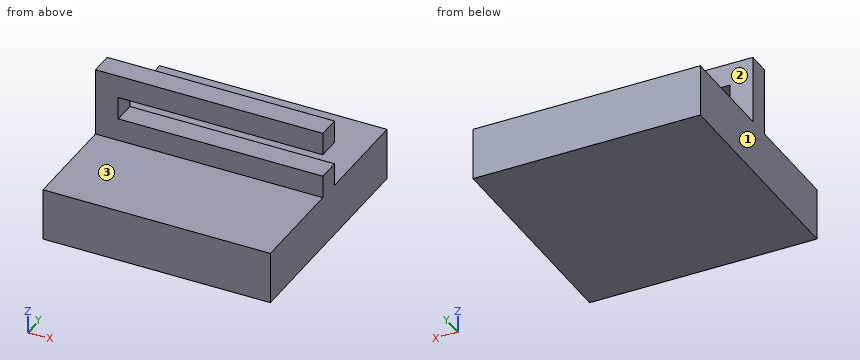
```python
from build123d import *

# Parameters (mm, degrees)
SKETCH1_W           = 100
SKETCH1_H           = 100
BOSS_EXTRUDE1_DEPTH = 23
SKETCH17_W          = 30
SKETCH17_H          = 10
BOSS_EXTRUDE2_DEPTH = 100
SKETCH18_W          = 90
SKETCH18_H          = 10
CUT_EXTRUDE1_DEPTH  = 126.833222958


with BuildPart() as part:
    # Sketch1 → Boss-Extrude1 (new body)
    with BuildSketch(Plane.XY):
        with Locations((50, 50)):
            Rectangle(SKETCH1_W, SKETCH1_H)
    extrude(amount=BOSS_EXTRUDE1_DEPTH)

    # Sketch17 → Boss-Extrude2 (add, through all)
    with BuildSketch(Plane(origin=(0, 0, 0), x_dir=(0, 0, -1), z_dir=(1, 0, 0))):
        with Locations((-38, 50)):
            Rectangle(SKETCH17_W, SKETCH17_H)
    extrude(amount=BOSS_EXTRUDE2_DEPTH)

    # Sketch18 → Cut-Extrude1 (cut, through all)
    with BuildSketch(Plane(origin=(0, 55, 0), x_dir=(1, 0, 0), z_dir=(0, 1, 0))):
        with Locations((55, -38)):
            Rectangle(SKETCH18_W, SKETCH18_H)
    extrude(amount=-CUT_EXTRUDE1_DEPTH, mode=Mode.SUBTRACT)


solid = part.part
```
Check sheet for the modelled part. Datum: model origin and axes. Units: mm. Face numbers are marked on the shaded views. A direction names the side the tool comes from. Give positions to 0.01 mm unless a question says otherwise; leave off trailing zeros. Write each loop counter-clockwise with the first axis right and the second up, starting at its lowest first coordinate (ties: lowest second). Pieces come first, ordered by that corner, then holes.
Item 1: Cross-section at B-B (y = 49). Enter the section's corners in (x, z), and give its area (3 significant figures).
Item 2: Cross-section at A-A (x = 20.5). Enter the section's corners in (y, z), and give its area (3 significant figures).
Item 3: Cross-section at C-C (z = 39). Enter the section's corners in (x, y).
Item 4: Gauge pin test, flat ends, axial feed: pin 1 (15 mm diameter, centred on x = 37, z = 42, fed in from -Y); pin 2 (22.5 mm diameter, centred on x = 61, y = 84, fed in from +Z); pin 3 (15 mm diameter, centred on x = 27.5, z = 36, fed in from +Y); pin 4 (5 mm diameter, centred on x = 51, z = 25, fed in from +Y). Record the tip position at first contact, or that the pin passes through.
Item 5: Cross-section at D-D (z = 26). Enter the section's corners in (x, y).
Item 6: Access from +Z, -Z, +X, -X, +Y, -Y to the whole of each face (thin tool, end or side, straight path). Record for the marked faces 1, 2 and 3.
Item 7: Scan lines: L1, parallel to Z at x = 20.5, y = 48.5; L2, parallel to Z at x = 32, y = 78; L3, parallel to Y at x = 52, z = 32.5. Record each from-to range of solid material in increasing order.
Report:
1. outline: (0, 0) - (100, 0) - (100, 33) - (10, 33) - (10, 43) - (100, 43) - (100, 53) - (0, 53) - close
1. area: 4,400 mm2
2. outline: (0, 0) - (100, 0) - (100, 23) - (55, 23) - (55, 33) - (45, 33) - (45, 23) - (0, 23) - close; (45, 43) - (55, 43) - (55, 53) - (45, 53) - close
2. area: 2,500 mm2
3. outline: (0, 45) - (10, 45) - (10, 55) - (0, 55) - close
4. pin 1: stops at y = 45
4. pin 2: stops at z = 23
4. pin 3: stops at y = 55
4. pin 4: stops at y = 100
5. outline: (0, 45) - (100, 45) - (100, 55) - (0, 55) - close
6. face 1: +Z, -Z, -X, +Y, -Y
6. face 2: +Z, +X, -X, +Y
6. face 3: +Z, +X, -X, -Y
7. L1: z = 0 to 33, 43 to 53
7. L2: z = 0 to 23
7. L3: y = 45 to 55
